Verification items for this drawing (mm, ordinates from the low corner). A direction names the side the tool comes from. Give positions to 0.01 mm unless a question says otherwise; leave off trailing zeros. Loops run counter-clockwise (first coordinate to the right, second up) from the corner with the lowest first, then second, coordinate; pieces in that order, holes last. Notation, with made-up numbers: (16, 79.25) -> (59, 79.25) arc R9 ccw to (59, 86.25) -> close; hole circle Ø11 at (-37.5, 60.25). An arc over 180 degrees is marked (long way). Answer as CSV lines item,"result". Start each with the question number.
(1) Material ranges on line 1 (X direction, y = 1.8, z = 10); line 2 (X direction, y = 3.9, z = 10); line 3 (Y direction, x = 8.75, z = 7.75), recorded low to high. Write a range as from..to.
(2) Section check C-C on y = 3.1. Enter the section's corners in (x, z).
(3) Access from +Z, -Z, +X, -X, +Y, -Y to the whole of each face (thin tool, end or side, straight path). Record for the marked faces 1 and 2.
(4) Section check D-D on z = 14.25. Enter the section's corners in (x, y).
(5) Section check B-B on x = 3.75. Enter the section's corners in (y, z).
(6) Section check A-A on z = 10. Enter the section's corners in (x, y), plus the area to 3 significant figures.
(7) Release check for a two-part mould opening along X. For the marked faces 3, 4 and 5 record: pulls with the +X half, pulls with the -X half, needs draft (parallel to the pull), parting line crosses it, or undercut.
(8) Gauge pin test, flat ends, axial feed: pin 1 Ø0.8 at (y, z) = (0.5, 14.5) entering from -X; pin 2 Ø2 at (x, z) = (0.5, 5.5) entering from -Y; pin 3 Ø3 at (y, z) = (4.5, 2) entering from +X; pin 4 Ø4.5 at (x, z) = (6, 10) entering from -Y. Record the tip position at first contact, or that the pin passes through.
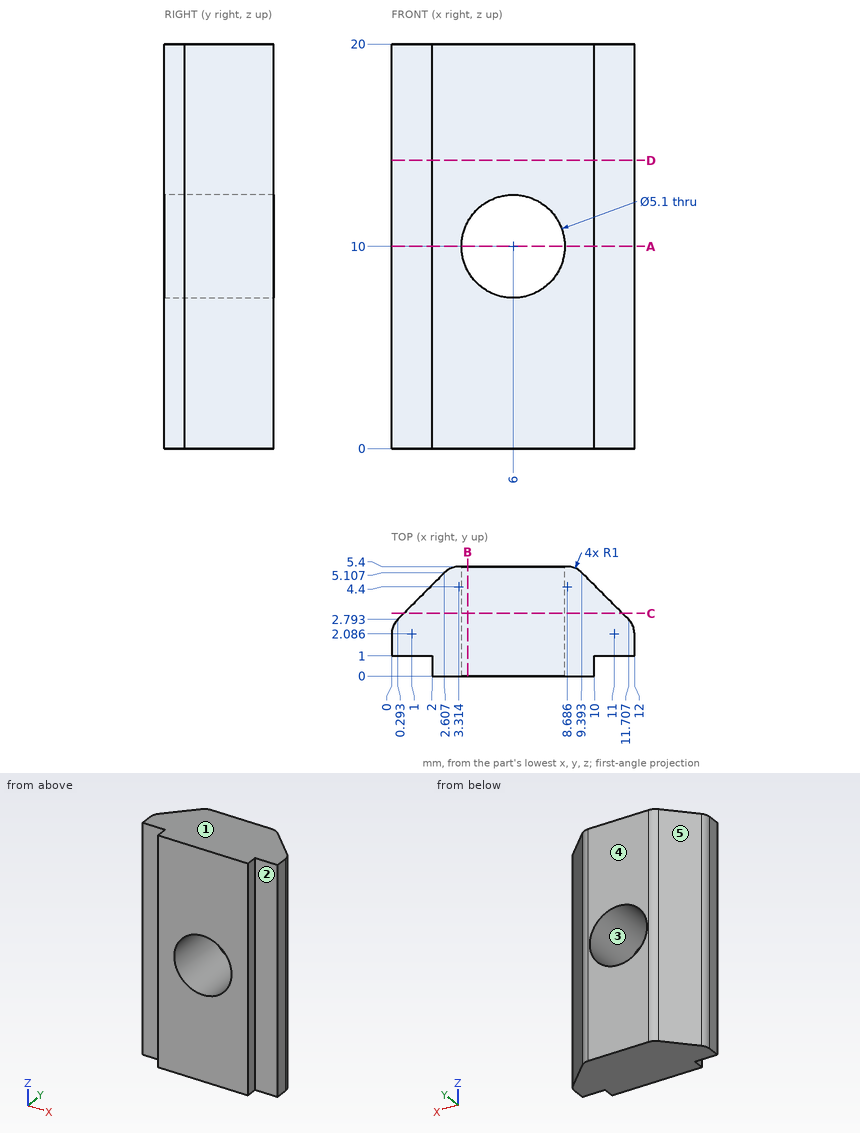
Working result:
1,line 1,"x = 0..3.45, 8.55..12"
1,line 2,"x = 1.4..3.45, 8.55..10.6"
1,line 3,"y = 0..5.4"
2,outline,"(0.6, 0) -> (11.4, 0) -> (11.4, 20) -> (0.6, 20) -> close; hole circle Ø5.1 at (6, 10)"
3,face 1,"+Z, +X, -X, +Y, -Y"
3,face 2,"+Z, -Z, +X, -Y"
4,outline,"(0, 1) -> (2, 1) -> (2, 0) -> (10, 0) -> (10, 1) -> (12, 1) -> (12, 2.09) arc R1 ccw to (11.71, 2.79) -> (9.39, 5.11) arc R1 ccw to (8.69, 5.4) -> (3.31, 5.4) arc R1 ccw to (2.61, 5.11) -> (0.29, 2.79) arc R1 ccw to (0, 2.09) -> close"
5,outline,"(0, 0) -> (5.4, 0) -> (5.4, 8.8) -> (0, 8.8) -> close; (0, 11.2) -> (5.4, 11.2) -> (5.4, 20) -> (0, 20) -> close"
6,outline,"(0, 1) -> (2, 1) -> (2, 0) -> (3.45, 0) -> (3.45, 5.4) -> (3.31, 5.4) arc R1 ccw to (2.61, 5.11) -> (0.29, 2.79) arc R1 ccw to (0, 2.09) -> close; (8.55, 0) -> (10, 0) -> (10, 1) -> (12, 1) -> (12, 2.09) arc R1 ccw to (11.71, 2.79) -> (9.39, 5.11) arc R1 ccw to (8.69, 5.4) -> (8.55, 5.4) -> close"
6,area,"24.8 mm^2"
7,face 3,"undercut"
7,face 4,"needs draft"
7,face 5,"pulls with the -X half"
8,pin 1,"stops at x = 2"
8,pin 2,"stops at y = 1"
8,pin 3,"stops at x = 11.5"
8,pin 4,"passes through"
